The figure shows three views and two pictorial views of one solid part (mm, origin at its lowest corner). Answer the questions. Round coordinates to 2 decimals unless told otherwise and drop trailing zeros. Write each loop counter-clockwise with the first axis right and the second up, starting at its lowest first coordinate (ties: lowest second). Pieces come first, ordered by that corner, then holes. Notation, with made-up numbers: M 10,29.25 L 39,29.25 A28 ccw 39,64.25 Z; hole C 35,69 d9. An arc over 180 degrees is marked long. One line per item, written item: value. Start each with the question number.
Q1. Find section A-A (x = 11). Write down the section's boundary in (y, z), and give its area (3 significant figures).
Q2. The mould has two halves that part along Y. Classify the marked faces 1, 2, 3 and 4: released by +Y, released by -Y, zero draft, split by the parting line, or undercut.
Q3. Find section B-B (z = 5). Write down the section's boundary in (x, y), and give its area (3 significant figures).
Q4. Find section D-D (y = 28). Write down the section's boundary in (x, z).
Q5. Given pin 1 Ø4 at (x, y) = (13, 24) entering from -Z; pin 2 Ø4 at (y, z) = (8.5, 3.5) entering from +X; pin 3 Ø3 at (y, z) = (18.5, 7) entering from +X, each flat-ended and moving along its own axis, determine where each tip first touches the part or whether it passes through.
Q6. Consider probe 1 along X at (y, z) = (20.5, 7); probe 2 along Y at (x, z) = (13.75, 8); probe 3 along Y at (x, z) = (17.25, 3.5). Determine where each line is inside the solid, lowest interval first.
Q7. Find section C-C (y = 9.5). Write down the section's boundary in (x, z), and give its area (3 significant figures).
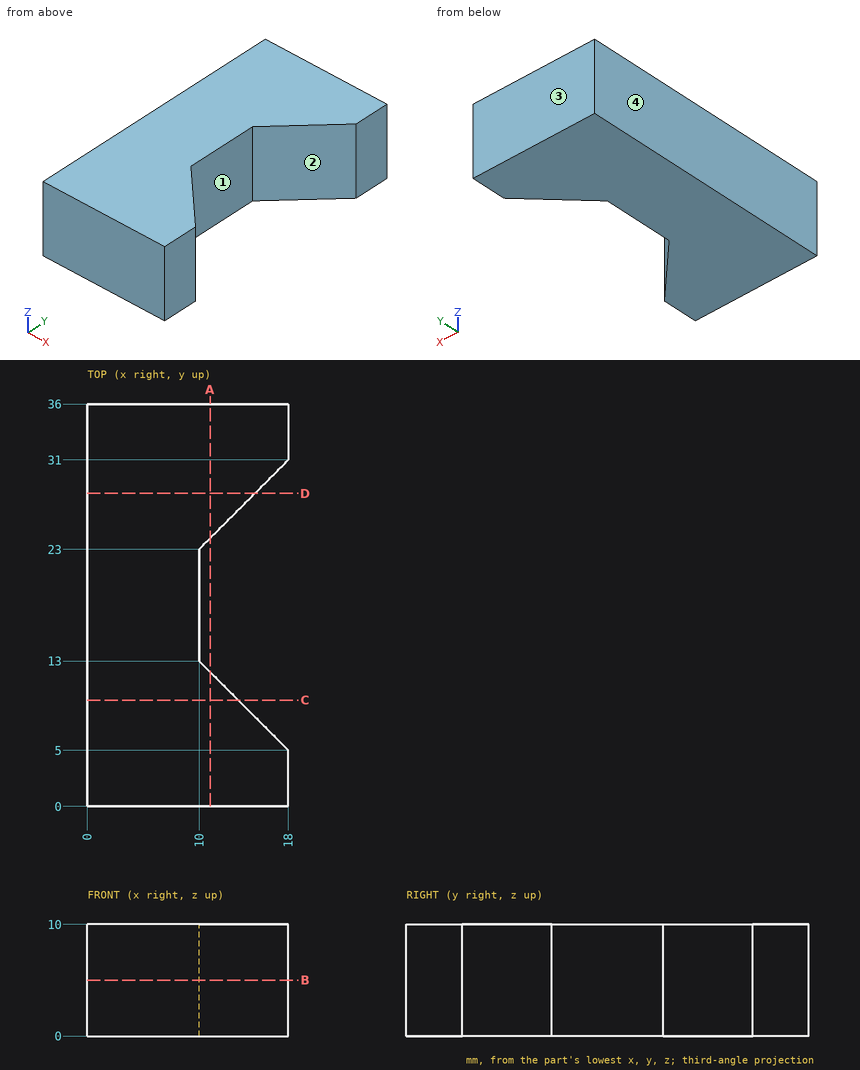
The answers:
1. outline: M 0,0 L 12,0 L 12,10 L 0,10 Z; M 24,0 L 36,0 L 36,10 L 24,10 Z
1. area: 240 mm2
2. face 1: undercut
2. face 2: undercut
2. face 3: released by +Y
2. face 4: zero draft
3. outline: M 0,0 L 18,0 L 18,5 L 10,13 L 10,23 L 18,31 L 18,36 L 0,36 Z
3. area: 504 mm2
4. outline: M 0,0 L 15,0 L 15,10 L 0,10 Z
5. pin 1: z = 0
5. pin 2: x = 16.5
5. pin 3: x = 10
6. probe 1: 0 to 10
6. probe 2: 0 to 9.25, 26.75 to 36
6. probe 3: 0 to 5.75, 30.25 to 36
7. outline: M 0,0 L 13.5,0 L 13.5,10 L 0,10 Z
7. area: 135 mm2
